Read the model definition and answer for the solid it produces. Units are mm, in the model's axes. A direction names the side the tool comes from. Round coordinates to 2 decimals unless told otherwise and drop trailing zeros. Order: outer loops, then holes, each group sorted by start corner. A loop starts at its lowest first (then second) coordinate and runs counter-clockwise, first axis right, second up. Notation, with made-up numbers: (42.5, -17.75) -> (66.5, -17.75) arc R33 cw to (66.5, 11.25) -> close; hole circle Ø11 at (12, 46.25). An arc over 180 degrees is marked (long way). Answer as a JSON object with one key per item and string values. Group by question number.
Item 1: Section B-B, the plane x = 33 is taken. Write down the section's boundary in (y, z).
Item 2: Section A-A, the plane x = 57.15 is taken. Write down the section's boundary in (y, z).
Item 3: The mould has two halves that part along Y. Classify faces 4 (the flat face through (35, 0, 13)), 5 (the cylindrical face through (7.66, -16.56, 6.44)), 6 (the flat face through (5, -13, 12.7)): pulls with the +Y half, pulls with the -Y half, needs draft (parallel to the pull), parting line crosses it, or undercut.
Item 4: For faces 1 (the cylindrical face through (31.928, -6.643, 33.657)), 2 (the flat face through (60.2, -6.9, 12.7)), 3 (the flat face through (19.05, -13, 25)), determine the directions among +Z, -Z, +X, -X, +Y, -Y from which every point of the face is accessible in a straight line to the end or side of a thin tool.
Item 5: Consider probe 1 along X at (y, z) = (-12.75, 10.5); probe 2 along X at (y, z) = (-13.25, 15.5); probe 3 along Z at (x, y) = (38, -12.7). Determine where each line is inside the solid, lowest interval first. Write a range as from..to.
Item 6: Given P1, Ø15, axis at x = 8, y = -15, coming from the +Z side; P2, Ø2, axis at y = -4.5, z = 31.5, coming from the -X side; P3, Ø3, axis at x = 40, y = -8, coming from the +Z side; P4, Ø3, axis at x = 56.5, y = -16.5, coming from the -Z side, each flat-ended and moving along its own axis, determine where each tip first touches the part or whether it passes through.
Item 7: Section D-D, the plane z = 34.5 is taken. Write down the section's boundary in (x, y).
Item 8: Section C-C, the plane y = -10.25 is taken. Write down the section's boundary in (x, z), plus the area to 3 significant figures.
from build123d import *

# Parameters (mm, degrees)
F1_DEPTH = 25.4
F2_R     = 6.35
F3_DEPTH = 25.4
F5_DEPTH = 25.4
F6_R     = 6.35
F7_DEPTH = 25.4


with BuildPart() as f1:
    # F0 (on Front) → F1 (new body)
    with BuildSketch(Plane.XZ):
        Polygon((0, 12.7), (0, 0), (69.85, 0), (69.85, 12.7), (44.45, 12.7), (44.45, 44.45), (19.05, 44.45), (19.05, 12.7), align=None)
    extrude(amount=F1_DEPTH)

    # F2 (on face) → F3 (cut)
    with BuildSketch(Plane.XY.offset(12.7)):
        with Locations((12.7, -12.7)):
            Circle(F2_R)
        with Locations((57.15, -12.7)):
            Circle(F2_R)
        with BuildLine():
            ThreePointArc((69.85, -12.7), (68.1740316571, -19.7995158286), (63.5, -25.4))
            Line((63.5, -25.4), (69.85, -25.4))
            Line((69.85, -25.4), (69.85, -12.7))
        make_face()
        with BuildLine():
            ThreePointArc((63.5, 0), (68.1740316571, -5.6004841714), (69.85, -12.7))
            Line((69.85, -12.7), (69.85, 0))
            Line((69.85, 0), (63.5, 0))
        make_face()
    extrude(amount=-F3_DEPTH, mode=Mode.SUBTRACT)

    # F4 (on face) → F5 (cut)
    with BuildSketch(Plane.XY.offset(12.7)):
        with BuildLine():
            ThreePointArc((0, -12.7), (1.6759683429, -5.6004841714), (6.35, 0))
            Line((6.35, 0), (0, 0))
            Line((0, 0), (0, -12.7))
        make_face()
        with BuildLine():
            ThreePointArc((6.35, -25.4), (1.6759683429, -19.7995158286), (0, -12.7))
            Line((0, -12.7), (0, -25.4))
            Line((0, -25.4), (6.35, -25.4))
        make_face()
    extrude(amount=-F5_DEPTH, mode=Mode.SUBTRACT)

    # F6 (on face) → F7 (cut)
    with BuildSketch(Plane.YZ.offset(44.45)):
        with BuildLine():
            ThreePointArc((-25.4, 31.75), (-12.7, 44.3458432454), (0, 31.75))
            Line((0, 31.75), (0, 44.45))
            Line((0, 44.45), (-25.4, 44.45))
            Line((-25.4, 44.45), (-25.4, 31.75))
        make_face()
        with Locations((-12.7, 31.75)):
            Circle(F6_R)
    extrude(amount=-F7_DEPTH, mode=Mode.SUBTRACT)


solid = f1.part
Values found:
{
 "1": {"outline": "(-25.4, 0) -> (0, 0) -> (0, 31.75) arc R12.7 ccw to (-25.4, 31.75) -> close; hole circle Ø12.7 at (-12.7, 31.75)"},
 "2": {"outline": "(-25.4, 0) -> (-19.05, 0) -> (-19.05, 12.7) -> (-25.4, 12.7) -> close; (-6.35, 0) -> (0, 0) -> (0, 12.7) -> (-6.35, 12.7) -> close"},
 "3": {"face 4": "pulls with the +Y half", "face 5": "undercut", "face 6": "needs draft"},
 "4": {"face 1": "+X, -X", "face 2": "+Z, +X, +Y, -Y", "face 3": "+Z, -X, +Y, -Y"},
 "5": {"probe 1": "0..6.35, 19.05..50.8, 63.5..69.85", "probe 2": "19.05..44.45", "probe 3": "0..25.4, 38.1..44.35"},
 "6": {"P1": "z = 12.7", "P2": "x = 19.05", "P3": "z = 43.94", "P4": "through"},
 "7": {"outline": "(19.05, -25.08) -> (44.45, -25.08) -> (44.45, -18.42) -> (19.05, -18.42) -> close; (19.05, -6.98) -> (44.45, -6.98) -> (44.45, -0.32) -> (19.05, -0.32) -> close"},
 "8": {"outline": "(0.19, 0) -> (6.84, 0) -> (6.84, 12.7) -> (0.19, 12.7) -> close; (18.56, 0) -> (51.29, 0) -> (51.29, 12.7) -> (44.45, 12.7) -> (44.45, 25.89) -> (19.05, 25.89) -> (19.05, 12.7) -> (18.56, 12.7) -> close; (19.05, 37.61) -> (44.45, 37.61) -> (44.45, 44.11) -> (19.05, 44.11) -> close; (63.01, 0) -> (69.66, 0) -> (69.66, 12.7) -> (63.01, 12.7) -> close", "area": "1,080 mm2"}
}
